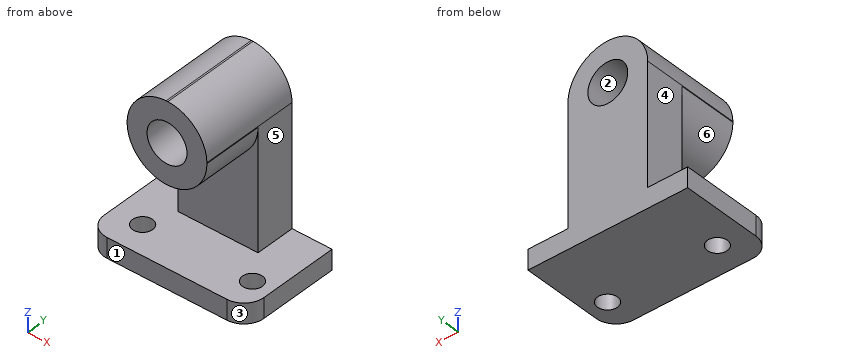
from build123d import *

# Parameters (mm, degrees)
F0_W      = 50.8
F0_H      = 57.15
F1_DEPTH  = 31.75
F2_W      = 12.7
F2_H      = 50.8
F3_DEPTH  = 31.75
F5_DEPTH  = 19.05
F7_DEPTH  = 31.75
F8_R      = 3.175
F9_DEPTH  = 6.35
F10_R     = 6.35
F11_DEPTH = 31.75


with BuildPart() as f1:
    # F0 (on Front) → F1 (new body)
    with BuildSketch(Plane.XZ):
        with Locations((25.4, 28.575)):
            Rectangle(F0_W, F0_H)
    extrude(amount=F1_DEPTH)

    # F2 (on face) → F3 (cut)
    with BuildSketch(Plane.XZ.offset(31.75)):
        with Locations((6.35, 31.75)):
            Rectangle(F2_W, F2_H)
        with Locations((44.45, 31.75)):
            Rectangle(F2_W, F2_H)
    extrude(amount=-F3_DEPTH, mode=Mode.SUBTRACT)

    # F4 (on face) → F5 (cut)
    with BuildSketch(Plane.XZ.offset(31.75)):
        with BuildLine():
            Line((12.7, 44.45), (12.7, 6.35))
            Line((12.7, 6.35), (38.1, 6.35))
            Line((38.1, 6.35), (38.1, 44.45))
            ThreePointArc((38.1, 44.45), (25.4, 31.75), (12.7, 44.45))
        make_face()
    extrude(amount=-F5_DEPTH, mode=Mode.SUBTRACT)

    # F6 (on face) → F7 (cut)
    with BuildSketch(Plane.XZ.offset(31.75)):
        with BuildLine():
            Line((12.7, 57.15), (12.7, 44.7116427085))
            ThreePointArc((12.7, 44.7116427085), (16.4178383196, 53.4321616804), (25.1383572915, 57.15))
            Line((25.1383572915, 57.15), (12.7, 57.15))
        make_face()
        with BuildLine():
            ThreePointArc((25.6616427085, 57.15), (34.3821616804, 53.4321616804), (38.1, 44.7116427085))
            Line((38.1, 44.7116427085), (38.1, 57.15))
            Line((38.1, 57.15), (25.6616427085, 57.15))
        make_face()
    extrude(amount=-F7_DEPTH, mode=Mode.SUBTRACT)

    # F8 (on face) → F9 (cut)
    with BuildSketch(Plane.XY.offset(6.35)):
        with Locations((9.525, -22.225)):
            Circle(F8_R)
        with BuildLine():
            ThreePointArc((6.35, -31.75), (1.8598719395, -29.8901280605), (0, -25.4))
            Line((0, -25.4), (0, -31.75))
            Line((0, -31.75), (6.35, -31.75))
        make_face()
        with Locations((44.45, -22.225)):
            Circle(F8_R)
        with BuildLine():
            ThreePointArc((50.8, -25.4), (48.9401280605, -29.8901280605), (44.45, -31.75))
            Line((44.45, -31.75), (50.8, -31.75))
            Line((50.8, -31.75), (50.8, -25.4))
        make_face()
    extrude(amount=-F9_DEPTH, mode=Mode.SUBTRACT)

    # F10 (on face) → F11 (cut)
    with BuildSketch(Plane.XZ.offset(31.75)):
        with Locations((25.4, 44.45)):
            Circle(F10_R)
    extrude(amount=-F11_DEPTH, mode=Mode.SUBTRACT)


solid = f1.part
The listing builds one solid part. Answer for the finished solid, in the listing's coordinates (mm). Face numbers are marked on the shaded views. A direction names the side the tool comes from. Coordinates: 2 decimals unless noted, no trailing zeros. Write each loop counter-clockwise with the first axis right and the second up, starting at its lowest first coordinate (ties: lowest second). Pieces come first, ordered by that corner, then holes. Notation, with made-up numbers: (-6, 68) -> (10, 68) arc R27 cw to (10, 98) -> close; hole circle Ø3 at (13.5, -25.5). An arc over 180 degrees is marked (long way). One line per question, with ' | ' between items.
1. Section B-B (x = 8.5) is taken. Determine the outline of the cut face in (y, z), and give its area (3 significant figures).
Verdict:
outline: (-31.75, 0) -> (-25.23, 0) -> (-25.23, 6.35) -> (-31.75, 6.35) -> close; (-19.22, 0) -> (0, 0) -> (0, 6.35) -> (-19.22, 6.35) -> close | area: 163 mm^2
2. Given pin 1 Ø9.5 at (y, z) = (-15, 19.5) entering from +X; pin 2 Ø16 at (y, z) = (-13.5, 27) entering from -X; pin 3 Ø4 at (x, z) = (19.5, 13.5) entering from -Y; pin 4 Ø5.5 at (x, y) = (44.45, -22.225) entering from -Z, each flat-ended and moving along its own axis, determine where each tip first touches the part or whether it passes through.
Verdict:
pin 1: stops at x = 38.1 | pin 2: stops at x = 12.7 | pin 3: stops at y = -12.7 | pin 4: passes through
3. Straight lines are drawn through the part: line 1 (Z direction, x = 25.4, y = -18.5); line 2 (Z direction, x = 25.4, y = -7.5); line 3 (X direction, y = -20, z = 2.5). For each, find the intervals that lie inside material, in ascending order.
Verdict:
line 1: z = 0 to 6.35, 31.75 to 38.1, 50.8 to 57.15 | line 2: z = 0 to 38.1, 50.8 to 57.15 | line 3: x = 0 to 7.26, 11.79 to 42.19, 46.71 to 50.8
4. Section C-C (y = -4.5) is taken. Determine the outline of the cut face in (x, z).
Verdict:
outline: (0, 0) -> (50.8, 0) -> (50.8, 6.35) -> (38.1, 6.35) -> (38.1, 44.71) arc R12.7 ccw to (25.66, 57.15) -> (25.14, 57.15) arc R12.7 ccw to (12.7, 44.71) -> (12.7, 6.35) -> (0, 6.35) -> close; hole circle Ø12.7 at (25.4, 44.45)
5. Which of the six approach directions +Z, -Z, +X, -X, +Y, -Y give full straight-line access (tool end or side, diameter ignored) to the marked faces 4, 5 and 6?
Verdict:
face 4: +Z, -X, +Y, -Y | face 5: +Z, +X, +Y, -Y | face 6: -Y
6. Section D-D (z = 16) is taken. Determine the outline of the cut face in (x, y), and give its area (3 significant figures).
Verdict:
outline: (12.7, -12.7) -> (38.1, -12.7) -> (38.1, 0) -> (12.7, 0) -> close | area: 323 mm^2
7. Section A-A (y = -15) is taken. Determine the outline of the cut face in (x, z), and give its area (3 significant figures).
Verdict:
outline: (0, 0) -> (50.8, 0) -> (50.8, 6.35) -> (0, 6.35) -> close; (12.7, 44.45) arc R12.7 ccw to (38.1, 44.45) -> (38.1, 44.71) arc R12.7 ccw to (25.66, 57.15) -> (25.14, 57.15) arc R12.7 ccw to (12.7, 44.71) -> close; hole circle Ø12.7 at (25.4, 44.45) | area: 703 mm^2
8. For a pull along X with two mould halves and no side action, classify the marked faces 1, 2 and 3 as released by +X, released by -X, zero draft, split by the parting line, or undercut.
Verdict:
face 1: zero draft | face 2: undercut | face 3: released by +X
